```python
from build123d import *

# Parameters (mm, degrees)
SKETCH_1_R          = 1.75
EXTRUDE_1_DEPTH     = 6
FILLET_2_R          = 4.25
SKETCH_2_R          = 7.5
CUT_EXTRUDE_1_DEPTH = 10


with BuildPart() as part:
    # 草图1 → 凸台-拉伸1 (new body)
    with BuildSketch(Plane(origin=(0, 0, 0), x_dir=(1, 0, 0), z_dir=(0, 1, 0))):
        with BuildLine():
            Line((-17.5, -34.505556242), (-17.5, 0))
            ThreePointArc((-17.5, 0), (0, 17.5), (17.5, 0))
            ThreePointArc((17.5, 0), (12.374368671, -12.374368671), (0, -17.5))
            Line((0, -17.5), (0, -28.5))
            ThreePointArc((0, -28.5), (-9.250901385, -30.043167405), (-17.5, -34.505556242))
        make_face()
        with Locations((0, 13.5)):
            Circle(SKETCH_1_R, mode=Mode.SUBTRACT)
        with Locations((11.691342951, 6.75)):
            Circle(SKETCH_1_R, mode=Mode.SUBTRACT)
        with Locations((11.691342951, -6.75)):
            Circle(SKETCH_1_R, mode=Mode.SUBTRACT)
        with Locations((0, -13.5)):
            Circle(SKETCH_1_R, mode=Mode.SUBTRACT)
        with Locations((-11.691342951, -6.75)):
            Circle(SKETCH_1_R, mode=Mode.SUBTRACT)
        with Locations((-11.691342951, 6.75)):
            Circle(SKETCH_1_R, mode=Mode.SUBTRACT)
    extrude(amount=EXTRUDE_1_DEPTH)

    # 圆角2
    fillet_2_edges = [part.edges().sort_by_distance(p)[0] for p in [
        (0, 3, 17.5),
    ]]
    fillet(fillet_2_edges, radius=FILLET_2_R)

    # 草图2 → 切除-拉伸1 (cut)
    with BuildSketch(Plane(origin=(0, 6, 0), x_dir=(1, 0, 0), z_dir=(0, 1, 0))):
        Circle(SKETCH_2_R)
    extrude(amount=-CUT_EXTRUDE_1_DEPTH, mode=Mode.SUBTRACT)


solid = part.part
```
Input: part model. Units: mm. Frame: model coordinates. Coordinates: 2 decimals unless noted, no trailing zeros. Loops run counter-clockwise (first coordinate to the right, second up) from the corner with the lowest first, then second, coordinate; pieces in that order, holes last.
Q1. Line query: line 1 along X through (y, z) = (2, -6.75); line 2 along X through (y, z) = (2.05, 6.75); line 3 along Z through (x, y) = (-11.5, 2.95). Output: solid intervals per line, ascending.
Results are:
line 1: x = -16.15 to -13.44, -9.94 to -3.27, 3.27 to 9.94, 13.44 to 16.15
line 2: x = -17.5 to -13.44, -9.94 to -3.27, 3.27 to 9.94, 13.44 to 16.15
line 3: z = -13.19 to -8.49, -5.01 to 5.01, 8.49 to 30.92
Q2. Section B-B, the plane x = -3.5. Return the cut outline in (y, z), and give its area (3 significant figures).
Results are:
outline: (0, -17.15) - (6, -17.15) - (6, -6.63) - (0, -6.63) - close; (0, 6.63) - (6, 6.63) - (6, 28.72) - (0, 28.72) - close
area: 196 mm2
Q3. Section A-A, the plane y = 0.9. Return the cut outline in (x, z).
Results are:
outline: (-17.5, 0) arc R17.5 ccw (long way) to (3.42, 17.16) arc R4.25 cw to (0, 21.33) - (0, 28.5) arc R28.5 cw to (-17.5, 34.51) - close; hole circle Ø3.5 at (-11.69, -6.75); hole circle Ø3.5 at (-11.69, 6.75); hole circle Ø15 at (0, 0); hole circle Ø3.5 at (0, -13.5); hole circle Ø3.5 at (0, 13.5); hole circle Ø3.5 at (11.69, -6.75); hole circle Ø3.5 at (11.69, 6.75)
Q4. Section D-D, the plane z = -3.5. Return the cut outline in (x, y).
Results are:
outline: (-17.15, 0) - (-6.63, 0) - (-6.63, 6) - (-17.15, 6) - close; (6.63, 0) - (17.15, 0) - (17.15, 6) - (6.63, 6) - close
Q5. Mould query, pull axis X, two halves, no side actions, for faces 1 (the flat face through (-4, 0, 8)), 2 (the cylindrical face through (13.31, 2.96, -6.08)), 3 (the flat face through (0, 3, 25)). Classes: +X half, -X half, draft (parallel to the pull), parting line (faces both ways), or undercut.
Results are:
face 1: draft
face 2: undercut
face 3: +X half
Q6. Section C-C, the plane z = 6.75. Return the cut outline in (x, y).
Results are:
outline: (-17.5, 0) - (-13.44, 0) - (-13.44, 6) - (-17.5, 6) - close; (-9.94, 0) - (-3.27, 0) - (-3.27, 6) - (-9.94, 6) - close; (3.27, 0) - (9.94, 0) - (9.94, 6) - (3.27, 6) - close; (13.44, 0) - (16.15, 0) - (16.15, 6) - (13.44, 6) - close
